Here's how the part is built. I have some questions about the finished solid (model axes, mm). A direction names the side the tool comes from. Round coordinates to 2 decimals unless told otherwise and drop trailing zeros. Loops run counter-clockwise (first coordinate to the right, second up) from the corner with the lowest first, then second, coordinate; pieces in that order, holes last. Notation, with made-up numbers: M 18,-9.5 L 37,-9.5 A11 cw 37,-4.5 Z; hole C 19,-25 d2. An arc over 180 degrees is marked long. Answer as a JSON object with one key per item and string values.
from build123d import *

# Parameters (mm, degrees)
CROQUIS1_R              = 10.8
CROQUIS1_R_2            = 2.7
SALIENTE_EXTRUIR1_DEPTH = 11.5
BOSS_EXTRUDE1_START     = 1
BOSS_EXTRUDE1_DEPTH     = 9.5


with BuildPart() as part:
    # Croquis1 → Saliente-Extruir1 (new body)
    with BuildSketch(Plane(origin=(0, 0, 0), x_dir=(1, 0, 0), z_dir=(0, 1, 0))):
        Circle(CROQUIS1_R)
        with Locations(Location((0, 0, 0), (0, 0, 270))):
            Circle(CROQUIS1_R_2, mode=Mode.SUBTRACT)
        with BuildLine():
            Line((13.3, 1.25), (10.563906891, 2.24585645))
            ThreePointArc((10.563906891, 2.24585645), (10.740814551, 1.129115932), (10.8, 0))
            ThreePointArc((10.8, 0), (10.740814551, -1.129115932), (10.563906891, -2.24585645))
            Line((10.563906891, -2.24585645), (13.3, -1.25))
            Line((13.3, -1.25), (13.3, 1.25))
        make_face()
        with BuildLine():
            Line((10.02519446, 8.828815098), (7.226298902, 8.026244712))
            ThreePointArc((7.226298902, 8.026244712), (8.737383539, 6.348080725), (9.866461502, 4.392372642))
            Line((9.866461502, 4.392372642), (11.494657591, 6.806272613))
            Line((11.494657591, 6.806272613), (10.02519446, 8.828815098))
        make_face()
        with BuildLine():
            Line((5.349828089, 10.8), (5.298746671, 12.262780424))
            Line((5.298746671, 12.262780424), (2.92110538, 13.03532291))
            Line((2.92110538, 13.03532291), (1.128490345, 10.740880296))
            ThreePointArc((1.128490345, 10.740880296), (3.337383539, 10.271410376), (5.400363168, 9.352864677))
            Line((5.400363168, 9.352864677), (5.349828089, 10.8))
        make_face()
        with BuildLine():
            ThreePointArc((-5.400363168, 9.352864677), (-3.337383539, 10.271410376), (-1.128490345, 10.740880296))
            Line((-1.128490345, 10.740880296), (-2.92110538, 13.03532291))
            Line((-2.92110538, 13.03532291), (-5.298746671, 12.262780424))
            Line((-5.298746671, 12.262780424), (-5.400363168, 9.352864677))
        make_face()
        with BuildLine():
            ThreePointArc((-9.866461502, 4.392372642), (-8.737383539, 6.348080725), (-7.226298902, 8.026244712))
            Line((-7.226298902, 8.026244712), (-10.02519446, 8.828815098))
            Line((-10.02519446, 8.828815098), (-11.494657591, 6.806272613))
            Line((-11.494657591, 6.806272613), (-9.866461502, 4.392372642))
        make_face()
        with BuildLine():
            ThreePointArc((-10.563906891, -2.24585645), (-10.8, 0), (-10.563906891, 2.24585645))
            Line((-10.563906891, 2.24585645), (-13.3, 1.25))
            Line((-13.3, 1.25), (-13.3, -1.25))
            Line((-13.3, -1.25), (-10.563906891, -2.24585645))
        make_face()
        with BuildLine():
            ThreePointArc((-7.226298902, -8.026244712), (-8.737383539, -6.348080725), (-9.866461502, -4.392372642))
            Line((-9.866461502, -4.392372642), (-11.494657591, -6.806272613))
            Line((-11.494657591, -6.806272613), (-10.02519446, -8.828815098))
            Line((-10.02519446, -8.828815098), (-7.226298902, -8.026244712))
        make_face()
        with BuildLine():
            ThreePointArc((-1.128490345, -10.740880296), (-3.337383539, -10.271410376), (-5.400363168, -9.352864677))
            Line((-5.400363168, -9.352864677), (-5.298746671, -12.262780424))
            Line((-5.298746671, -12.262780424), (-2.92110538, -13.03532291))
            Line((-2.92110538, -13.03532291), (-1.128490345, -10.740880296))
        make_face()
        with BuildLine():
            Line((5.298746671, -12.262780424), (5.400363168, -9.352864677))
            ThreePointArc((5.400363168, -9.352864677), (3.337383539, -10.271410376), (1.128490345, -10.740880296))
            Line((1.128490345, -10.740880296), (2.92110538, -13.03532291))
            Line((2.92110538, -13.03532291), (5.298746671, -12.262780424))
        make_face()
        with BuildLine():
            Line((11.494657591, -6.806272613), (9.866461502, -4.392372642))
            ThreePointArc((9.866461502, -4.392372642), (8.737383539, -6.348080725), (7.226298902, -8.026244712))
            Line((7.226298902, -8.026244712), (10.02519446, -8.828815098))
            Line((10.02519446, -8.828815098), (11.494657591, -6.806272613))
        make_face()
    extrude(amount=SALIENTE_EXTRUIR1_DEPTH)

    # Croquis1<6> → Boss-Extrude1 (add)
    with BuildSketch(Plane(origin=(0, 0, 0), x_dir=(1, 0, 0), z_dir=(0, 1, 0)).offset(BOSS_EXTRUDE1_START)):
        with BuildLine():
            Line((29.025420212, 10.8), (5.349828089, 10.8))
            Line((5.349828089, 10.8), (5.400363168, 9.352864677))
            ThreePointArc((5.400363168, 9.352864677), (6.348080725, 8.737383539), (7.226298902, 8.026244712))
            Line((7.226298902, 8.026244712), (10.02519446, 8.828815098))
            Line((10.02519446, 8.828815098), (11.494657591, 6.806272613))
            Line((11.494657591, 6.806272613), (9.866461502, 4.392372642))
            ThreePointArc((9.866461502, 4.392372642), (10.271410376, 3.337383539), (10.563906891, 2.24585645))
            Line((10.563906891, 2.24585645), (13.3, 1.25))
            Line((13.3, 1.25), (13.3, -1.25))
            Line((13.3, -1.25), (10.563906891, -2.24585645))
            ThreePointArc((10.563906891, -2.24585645), (10.512933542, -2.473505273), (10.457055035, -2.7))
            Line((10.457055035, -2.7), (19.42731544, -2.7))
            ThreePointArc((19.42731544, -2.7), (20.625475176, -3.098621454), (21.346022736, -4.135586754))
            ThreePointArc((21.346022736, -4.135586754), (52.452433734, -22.022808697), (71.724168494, 8.245355326))
            ThreePointArc((71.724168494, 8.245355326), (71.219997226, 8.647854219), (70.738687337, 8.218279059))
            ThreePointArc((70.738687337, 8.218279059), (50.52963152, -8.979070796), (31.015135616, 9.002565078))
            ThreePointArc((31.015135616, 9.002565078), (30.36610471, 10.284104133), (29.025420212, 10.8))
        make_face()
    extrude(amount=BOSS_EXTRUDE1_DEPTH)


solid = part.part
Item 1: I'm going to push flat-ended pins straight in: pin 1 Ø1 at (x, y) = (-1, 8) entering from -Z; pin 2 Ø4 at (y, z) = (9.5, 13) entering from +X; pin 3 Ø1 at (x, z) = (28.5, 4.5) entering from +Y. Where does each tip first touch, or does it pass through?
Resolved:
{"pin 1": "z = -11.22", "pin 2": "x = 68", "pin 3": "y = 10.5"}
Item 2: If we mould it in two halves opening along X, with no side actions, what happens to faces 1 (the face through (0, 0, 3)), 2 (the face through (-8.645, 5.67, 8.433)), 3 (the face through (-4.093, 5.67, -12.654)), 4 (the face through (10.77, 0.493, -7.803))? For each: pulls with the +X half, pulls with the -X half, needs draft (parallel to the pull), parting line crosses it, or undercut.
Resolved:
{"face 1": "needs draft", "face 2": "undercut", "face 3": "pulls with the -X half", "face 4": "pulls with the +X half"}
Item 3: On a 3-axis mill with a long thin cutter (end or side, diameter ignored), from which of +Z, -Z, +X, -X, +Y, -Y can I reach the whole of each face in a straight line? I mean faces 5 (the face through (6.335, 5.67, 8.747)), 6 (the face through (10.692, 5.67, 5.616)), 7 (the face through (2.037, 5.67, -11.904)), 8 (the face through (-10.75, 5.67, -7.83)), 9 (the face through (-10.276, 5.67, 3.322)). Say none if no direction works.
Resolved:
{"face 5": "+Z, +Y, -Y", "face 6": "+Y, -Y", "face 7": "-Z, +Y, -Y", "face 8": "-Z, -X, +Y, -Y", "face 9": "-X, +Y, -Y"}
Item 4: I want a section at A-A, the plane x = 0. Please give me the cut outline in (y, z).
Resolved:
{"outline": "M 0,-10.8 L 11.5,-10.8 L 11.5,-2.7 L 0,-2.7 Z; M 0,2.7 L 11.5,2.7 L 11.5,10.8 L 0,10.8 Z"}
Item 5: I want a section at B-B, the plane z = 0. Please give me the cut outline in (x, y).
Resolved:
{"outline": "M -13.3,0 L -2.7,0 L -2.7,11.5 L -13.3,11.5 Z; M 2.7,0 L 13.3,0 L 13.3,1 L 34.23,1 L 34.23,10.5 L 13.3,10.5 L 13.3,11.5 L 2.7,11.5 Z; M 67.62,1 L 72.02,1 L 72.02,10.5 L 67.62,10.5 Z"}
Item 6: Please list where these lines run through material, in increasing order: probe 1 along X at (y, z) = (6.25, 0); probe 2 along X at (y, z) = (8.25, -6); probe 3 along Y at (x, z) = (19.5, -1). Write a range as from..to.
Resolved:
{"probe 1": "-13.3..-2.7, 2.7..34.23, 67.62..72.02", "probe 2": "-10.95..31.55, 70.29..72.07", "probe 3": "1..10.5"}
Item 7: I want a section at C-C, the plane x = 66. Please give me the cut outline in (y, z), then the cut area to 3 significant figures.
Resolved:
{"outline": "M 1,2.13 L 10.5,2.13 L 10.5,13.67 L 1,13.67 Z", "area": "110 mm²"}
